```python
from build123d import *

# Parameters (mm, degrees)
IZIM2_R                     = 0.5
Y_KSEKLIK_EKSTR_ZYON1_DEPTH = 84
RADYUS1_R                   = 0.5
RADYUS4_R                   = 0.5


with BuildPart() as part:
    # Çizim2 → Yükseklik-Ekstrüzyon1 (new body)
    with BuildSketch(Plane(origin=(0, 0, 0), x_dir=(1, 0, 0), z_dir=(0, 1, 0))):
        Circle(IZIM2_R)
    extrude(amount=Y_KSEKLIK_EKSTR_ZYON1_DEPTH)

    # Radyus1
    radyus1_edges = [part.edges().sort_by_distance(p)[0] for p in [
        (-0.5, 84, 0),
    ]]
    fillet(radyus1_edges, radius=RADYUS1_R)

    # Radyus4
    radyus4_edges = [part.edges().sort_by_distance(p)[0] for p in [
        (-0.5, 0, 0),
    ]]
    fillet(radyus4_edges, radius=RADYUS4_R)


solid = part.part
```
The listing builds one solid part. Answer for the finished solid, in the listing's coordinates (mm). Coordinates: 2 decimals unless noted, no trailing zeros. Write each loop counter-clockwise with the first axis right and the second up, starting at its lowest first coordinate (ties: lowest second). Pieces come first, ordered by that corner, then holes. Notation, with made-up numbers: (11.5, 49.5) - (25.5, 49.5) arc R16 cw to (25.5, 61.5) - close; hole circle Ø5 at (-11, 51.5). An arc over 180 degrees is marked (long way). One line per item, written item: value.
1) Find section B-B (x = 0.35). Give the vertices of the cut face in (y, z), and give its area (3 significant figures).
Geometry check:
outline: (0.5, -0.36) - (83.5, -0.36) arc R0.36 ccw to (83.5, 0.36) - (0.5, 0.36) arc R0.36 ccw to start
area: 59.7 mm2
2) Find section A-A (y = 71). Give the vertices of the cut face in (x, z).
Geometry check:
outline: circle Ø1 at (0, 0)
3) Consider line 1 along Z through (x, y) = (-0.1, 68); line 2 along X through (y, z) = (17, -0.05); line 3 along Y through (x, z) = (0.3, 0.15). Determine where each line is inside the solid, lowest interval first. Write a range as from..to.
Geometry check:
line 1: z = -0.49..0.49
line 2: x = -0.5..0.5
line 3: y = 0.13..83.87
